Can you work these out from the model? Positions are in its coordinate system, mm. Face numbers are marked on the shaded views. Coordinates: 2 decimals unless noted, no trailing zeros. Order: outer loops, then holes, each group sorted by start corner. A loop starts at its lowest first (then second) coordinate and runs counter-clockwise, first axis right, second up. Notation, with made-up numbers: (-30, 14) -> (-16, 14) arc R21 ccw to (-16, 41) -> close; hole circle Ø5 at (51, -1.5). An arc over 180 degrees is marked (long way). Write item = value, one per line.
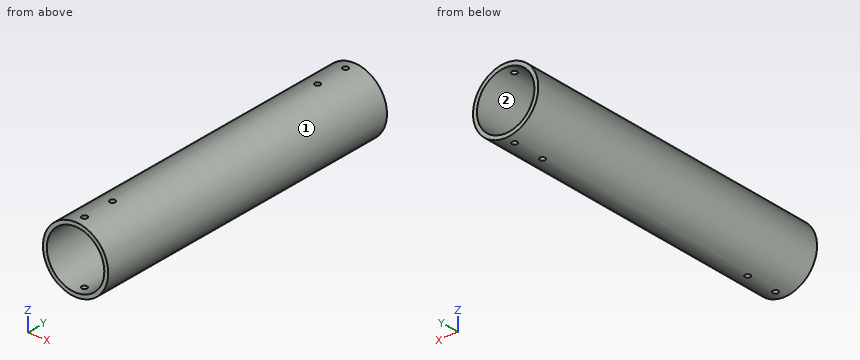
```python
from build123d import *

# Parameters (mm, degrees)
SKETCH_1_R          = 25
SKETCH_1_R_2        = 22
EXTRUDE_1_DEPTH     = 250
SKETCH_6_R          = 2.1
CUT_EXTRUDE_2_DEPTH = 30


with BuildPart() as part:
    # 草图1 → 拉伸-薄壁1 (new body)
    with BuildSketch(Plane(origin=(0, 0, 0), x_dir=(1, 0, 0), z_dir=(0, 1, 0))):
        Circle(SKETCH_1_R)
        Circle(SKETCH_1_R_2, mode=Mode.SUBTRACT)
    extrude(amount=EXTRUDE_1_DEPTH)

    # 草图6 → 切除-拉伸2 (cut, symmetric)
    with BuildSketch(Plane.XY):
        with Locations((0, 242)):
            Circle(SKETCH_6_R)
        with Locations((0, 8)):
            Circle(SKETCH_6_R)
        with Locations((0, 217)):
            Circle(SKETCH_6_R)
        with Locations((0, 33)):
            Circle(SKETCH_6_R)
    extrude(amount=CUT_EXTRUDE_2_DEPTH, both=True, mode=Mode.SUBTRACT)


solid = part.part
```
Item 1: I want a section at D-D, the plane y = 208. Please give me the cut outline in (x, z), plus the area to 3 significant figures.
A:
outline = circle Ø50 at (0, 0); hole circle Ø44 at (0, 0)
area = 443 mm2
Item 2: I'm going to push flat-ended pins straight in: P1, Ø10, axis at x = -8, y = 82, coming from the -Z side; P2, Ø3, axis at x = -6, y = 83, coming from the +Z side; P3, Ø2, axis at y = 67.5, z = -17, coming from the +X side; P4, Ø2.5, axis at x = 0, y = 33, coming from the +Z side. Where does each tip first touch, or does it pass through?
A:
P1 = -24.82
P2 = 24.59
P3 = 19.21
P4 = through
Item 3: I want a section at A-A, the plane z = 0. Please give me the cut outline in (x, y), plus the area to 3 significant figures.
A:
outline = (-25, 0) -> (-22, 0) -> (-22, 250) -> (-25, 250) -> close; (22, 0) -> (25, 0) -> (25, 250) -> (22, 250) -> close
area = 1,500 mm2
Item 4: I want a section at C-C, the plane x = 0. Give the number of separate pieces and of enclosed holes in the cut face, plus the area to 3 significant figures.
A:
separate_pieces = 10
enclosed_holes = 0
area = 1,400 mm2
Item 5: If I drill on probe 1 along Y at (x, z) = (0, 23); probe 2 along X at (y, z) = (175, 0.5) (3 decimals); probe 3 along Z at (x, y) = (0, 60), over which ranges is the centre line in solid material (lowest first)?
A:
probe_1 = 0 to 5.9, 10.1 to 30.9, 35.1 to 214.9, 219.1 to 239.9, 244.1 to 250
probe_2 = -24.995 to -21.994, 21.994 to 24.995
probe_3 = -25 to -22, 22 to 25
Item 6: If we mould it in two halves opening along X, with no side actions, what happens to the marked faces 1 and 2? For each: pulls with the +X half, pulls with the -X half, needs draft (parallel to the pull), parting line crosses it, or undercut.
A:
face_1 = parting line crosses it
face_2 = undercut
Item 7: I want a section at B-B, the plane x = 10. Please give me the cut outline in (y, z), plus the area to 3 significant figures.
A:
outline = (0, -22.91) -> (250, -22.91) -> (250, -19.6) -> (0, -19.6) -> close; (0, 19.6) -> (250, 19.6) -> (250, 22.91) -> (0, 22.91) -> close
area = 1,660 mm2
